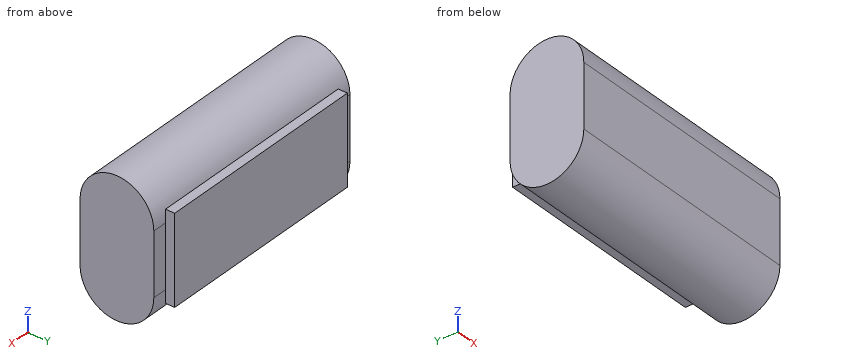
from build123d import *

# Parameters (mm, degrees)
EXTRUDE_1_DEPTH = 33.5
SKETCH_2_W      = 59
SKETCH_2_H      = 24
EXTRUDE_2_DEPTH = 2.5


with BuildPart() as part:
    # 草图1 → 凸台-拉伸1 (new, symmetric)
    with BuildSketch(Plane(origin=(0, 0, 0), x_dir=(0, 0, -1), z_dir=(1, 0, 0))):
        with BuildLine():
            Line((-8.5, 10), (8.5, 10))
            ThreePointArc((8.5, 10), (18.5, 0), (8.5, -10))
            Line((8.5, -10), (-8.5, -10))
            ThreePointArc((-8.5, -10), (-18.5, 0), (-8.5, 10))
        make_face()
    extrude(amount=EXTRUDE_1_DEPTH, both=True)

    # 草图2 → 凸台-拉伸2 (add)
    with BuildSketch(Plane(origin=(0, 10, 0), x_dir=(1, 0, 0), z_dir=(0, 1, 0))):
        Rectangle(SKETCH_2_W, SKETCH_2_H)
    extrude(amount=EXTRUDE_2_DEPTH)


solid = part.part
For this review, take the finished solid that the model builds, in its own axes (mm). Give positions to 0.01 mm unless a question says otherwise; leave off trailing zeros. Write each loop counter-clockwise with the first axis right and the second up, starting at its lowest first coordinate (ties: lowest second). Pieces come first, ordered by that corner, then holes. Notation, with made-up numbers: (19, 31) -> (34, 31) arc R23 cw to (34, 70) -> close; hole circle Ø7 at (36.25, -13). An arc over 180 degrees is marked (long way). Use CSV: the item, a comma, the result in double quotes.
Q1. To check wall thickness, follow probe 1 along Y at (x, z) = (30, 5); probe 2 along Y at (x, z) = (8.5, -16.5); probe 3 along Z at (x, y) = (3, 7.75). State the ranges of each line that lie inside material, in increasing order. Write a range as [from, to].
Conclusion:
probe 1,"[-10, 10]"
probe 2,"[-6, 6]"
probe 3,"[-14.82, 14.82]"
Q2. Take a section at C-C, the plane y = -6.25. Write out the cut boundary in (x, z).
Conclusion:
outline,"(-33.5, -16.31) -> (33.5, -16.31) -> (33.5, 16.31) -> (-33.5, 16.31) -> close"
Q3. Take a section at A-A, the plane x = -17. Write out the cut boundary in (y, z), then the cut area to 3 significant figures.
Conclusion:
outline,"(-10, -8.5) arc R10 ccw to (10, -8.5) -> (10, -12) -> (12.5, -12) -> (12.5, 12) -> (10, 12) -> (10, 8.5) arc R10 ccw to (-10, 8.5) -> close"
area,"714 mm2"
Q4. For P1, Ø6, axis at x = -2.5, y = 6, coming from the -Z side; P2, Ø3, axis at x = 5, y = 11, coming from the -Z side; P3, Ø2, axis at x = 16.5, y = 4.5, coming from the -Z side, all flat-tipped, find the tip position at first contact; note any pin that passes through.
Conclusion:
P1,"z = -18.04"
P2,"z = -12"
P3,"z = -17.87"
Q5. Take a section at B-B, the plane z = 15.5. Write out the cut boundary in (x, y).
Conclusion:
outline,"(-33.5, -7.14) -> (33.5, -7.14) -> (33.5, 7.14) -> (-33.5, 7.14) -> close"
